Design review of the part built by this model. Coordinates are the model's own, in mm. A direction names the side the tool comes from. Give positions to 0.01 mm unless a question says otherwise; leave off trailing zeros. Order: outer loops, then holes, each group sorted by start corner. A loop starts at its lowest first (then second) coordinate and runs counter-clockwise, first axis right, second up.
```python
from build123d import *

# Parameters (mm, degrees)
ESBO_O2_W                = 50
ESBO_O2_H                = 70
RESSALTO_EXTRUS_O1_DEPTH = 8
ESBO_O3_R                = 0.75
CORTE_EXTRUS_O1_DEPTH    = 30
FILETE1_R                = 2
ESBO_O17_W               = 10
ESBO_O17_H               = 5
RESSALTO_EXTRUS_O4_DEPTH = 8
ESBO_O20_R               = 2
CORTE_EXTRUS_O9_DEPTH    = 8
FILETE2_R                = 2.5
FILETE3_R                = 2.5
FILETE4_R                = 2.5
FILETE5_R                = 2.5
ESBO_O21_W               = 5
ESBO_O21_H               = 20
CORTE_EXTRUS_O10_DEPTH   = 9
FILETE6_R                = 2.5
ESBO_O22_R               = 1.5
CORTE_EXTRUS_O11_DEPTH   = 20


with BuildPart() as part:
    # Esboço2 → Ressalto-extrusão1 (new body)
    with BuildSketch(Plane.XY):
        with Locations((-42.281248797, -0.107598663)):
            Rectangle(ESBO_O2_W, ESBO_O2_H)
    extrude(amount=RESSALTO_EXTRUS_O1_DEPTH)

    # Esboço3 → Corte-extrusão1 (cut)
    with BuildSketch(Plane(origin=(0, -35.107598663, 0), x_dir=(-1, 0, 0), z_dir=(0, -1, 0))):
        with Locations((58.281248797, -4)):
            Circle(ESBO_O3_R)
        with Locations((63.281248797, -4)):
            Circle(ESBO_O3_R)
    extrude(amount=-CORTE_EXTRUS_O1_DEPTH, mode=Mode.SUBTRACT)

    # Filete1
    filete1_edges = [part.edges().sort_by_distance(p)[0] for p in [
        (-17.281248797, -0.107598663, 8),
    ]]
    fillet(filete1_edges, radius=FILETE1_R)

    # Esboço17 → Ressalto-extrusão4 (add)
    with BuildSketch(Plane(origin=(0, 0, 0), x_dir=(-1, 0, 0), z_dir=(0, 0, -1))):
        with Locations((72.281248797, -32.607598663)):
            Rectangle(ESBO_O17_W, ESBO_O17_H)
    extrude(amount=-RESSALTO_EXTRUS_O4_DEPTH)

    # Esboço20 → Corte-extrusão9 (cut)
    with BuildSketch(Plane.XZ.offset(35.107598663)):
        with Locations((-73.951248797, 4)):
            Circle(ESBO_O20_R)
    extrude(amount=-CORTE_EXTRUS_O9_DEPTH, mode=Mode.SUBTRACT)

    # Filete2
    filete2_edges = [part.edges().sort_by_distance(p)[0] for p in [
        (-67.281248797, 2.392401337, 8),
    ]]
    fillet(filete2_edges, radius=FILETE2_R)

    # Filete3
    filete3_edges = [part.edges().sort_by_distance(p)[0] for p in [
        (-67.281248797, 2.392401337, 0),
    ]]
    fillet(filete3_edges, radius=FILETE3_R)

    # Filete4
    filete4_edges = [part.edges().sort_by_distance(p)[0] for p in [
        (-77.281248797, -32.607598663, 8),
    ]]
    fillet(filete4_edges, radius=FILETE4_R)

    # Filete5
    filete5_edges = [part.edges().sort_by_distance(p)[0] for p in [
        (-77.281248797, -32.607598663, 0),
    ]]
    fillet(filete5_edges, radius=FILETE5_R)

    # Esboço21 → Corte-extrusão10 (cut, through all)
    with BuildSketch(Plane.XY.offset(8)):
        with Locations((-24.781248797, 18.892401337)):
            Rectangle(ESBO_O21_W, ESBO_O21_H)
        with Locations((-24.781248797, -19.107598663)):
            Rectangle(ESBO_O21_W, ESBO_O21_H)
    extrude(amount=-CORTE_EXTRUS_O10_DEPTH, mode=Mode.SUBTRACT)

    # Filete6
    filete6_edges = [part.edges().sort_by_distance(p)[0] for p in [
        (-17.281248797, -0.107598663, 0),
    ]]
    fillet(filete6_edges, radius=FILETE6_R)

    # Esboço22 → Corte-extrusão11 (cut)
    with BuildSketch(Plane(origin=(-17.281248797, 0, 0), x_dir=(0, 0, -1), z_dir=(1, 0, 0))):
        with Locations((-5, -25.107598663)):
            Circle(ESBO_O22_R)
        with Locations((-5, -14.107598663)):
            Circle(ESBO_O22_R)
        with Locations((-5, 24.892401337)):
            Circle(ESBO_O22_R)
        with Locations((-5, 13.892401337)):
            Circle(ESBO_O22_R)
    extrude(amount=-CORTE_EXTRUS_O11_DEPTH, mode=Mode.SUBTRACT)


solid = part.part
```
1. Draft analysis for pull direction X (two halves, no side actions). For faces 1 (the face through (-58.627, -20.318, 4.665)), 2 (the face through (-43, 34.892, 4)), 3 (the face through (-77.281, -33, 4)), state which applies: pulls with the +X half, pulls with the -X half, needs draft (parallel to the pull), parting line crosses it, or undercut.
Recorded:
face 1: undercut
face 2: needs draft
face 3: pulls with the -X half
2. Take a section at A-A (y = -20). State the section outline as (x, z) points, then the cut area to 3 significant figures.
Recorded:
outline: (-67.28, 2.5) arc R2.5 ccw to (-64.78, 0) - (-27.28, 0) - (-27.28, 8) - (-64.78, 8) arc R2.5 ccw to (-67.28, 5.5) - close; (-22.28, 0) - (-19.78, 0) arc R2.5 ccw to (-17.28, 2.5) - (-17.28, 6) arc R2 ccw to (-19.28, 8) - (-22.28, 8) - close; hole circle Ø1.5 at (-63.28, 4); hole circle Ø1.5 at (-58.28, 4)
area: 352 mm2
3. For line 1 along Y through (x, z) = (-21.3, 5); line 2 along X through (y, z) = (18.5, 3); line 3 along Y through (x, z) = (-73, 0.75), list the stretches that pass through material, from the lowest coordinate up.
Recorded:
line 1: y = -35.11 to -26.61, -23.61 to -15.61, -12.61 to 12.39, 15.39 to 23.39, 26.39 to 34.89
line 2: x = -67.28 to -27.28, -22.28 to -17.28
line 3: y = -35.11 to -30.11
4. Take a section at C-C (x = -30). State the section outline as (y, z) points.
Recorded:
outline: (-35.11, 0) - (34.89, 0) - (34.89, 8) - (-35.11, 8) - close; hole circle Ø3 at (-25.11, 5); hole circle Ø3 at (-14.11, 5); hole circle Ø3 at (13.89, 5); hole circle Ø3 at (24.89, 5)
5. Take a section at D-D (y = 2). State the section outline as (x, z) points.
Recorded:
outline: (-67.28, 2.5) arc R2.5 ccw to (-64.78, 0) - (-19.78, 0) arc R2.5 ccw to (-17.28, 2.5) - (-17.28, 6) arc R2 ccw to (-19.28, 8) - (-64.78, 8) arc R2.5 ccw to (-67.28, 5.5) - close
6. For pin 1 (1.8 mm diameter, centred on y = 24.89, z = 5, fed in from +X); pin 2 (2.5 mm diameter, centred on y = -25.11, z = 5, fed in from -X); pin 3 (1.5 mm diameter, centred on y = 17, z = 7, fed in from +X), all flat-tipped, find the tip position at first contact; note any pin that passes through.
Recorded:
pin 1: stops at x = -37.28
pin 2: stops at x = -67.28
pin 3: stops at x = -17.3
7. Take a section at B-B (y = 27.5). State the section outline as (x, z) points, then the cut area to 3 significant figures.
Recorded:
outline: (-67.28, 2.5) arc R2.5 ccw to (-64.78, 0) - (-27.28, 0) - (-27.28, 8) - (-64.78, 8) arc R2.5 ccw to (-67.28, 5.5) - close; (-22.28, 0) - (-19.78, 0) arc R2.5 ccw to (-17.28, 2.5) - (-17.28, 6) arc R2 ccw to (-19.28, 8) - (-22.28, 8) - close
area: 355 mm2
8. Machinability: for faces 4 (the face through (-58, -5.108, 4)), 5 (the face through (-37.281, 14, 5)), 6 (the face through (-22.281, 19, 4)), 7 (the face through (-66.529, 2.847, 7.287)), which of the approach directions +Z, -Z, +X, -X, +Y, -Y give a long, thin tool a straight path to every point of the face, cutting with its end or side? Answer none if there is none.
Recorded:
face 4: -Y
face 5: +X
face 6: +Z, -Z
face 7: +Z, -X, +Y
